Autodesk Inventor part; units mm, degrees
ref_plane "YZ Plane" through (0, 0, 0) normal (1, 0, 0) x (0, 1, 0)
ref_plane "XZ Plane" through (0, 0, 0) normal (0, 1, 0) x (-1, 0, 0)
ref_plane "XY Plane" through (0, 0, 0) normal (0, 0, 1) x (1, 0, 0)
sketch "スケッチ1" plane through (0, 0, 0) normal (1, 0, 0) x (0, 1, 0)
  line L0 (0, 0) -> (0, 6)
  line L1 (0, 6) -> (0, -6)
  line L2 (0, 0) -> (11.5, 0)
  line L3 (11.5, 0) -> (11.5, 9.5)
  line L4 (11.5, 9.5) -> (11.5, -9.5)
  circle A0 centre (0, 6) radius 1.25
  circle A1 centre (0, -6) radius 1.25
  circle A2 centre (11.5, 9.5) radius 1.65
  circle A3 centre (11.5, -9.5) radius 1.65
  circle A4 centre (11.5, 9.5) radius 2.5
  circle A5 centre (11.5, -9.5) radius 2.5
  circle A6 centre (0, 0) radius 2.65
  line L5 (0, 0) -> (-14.6, 0)
  circle A7 centre (-14.6, 0) radius 1.65
  circle A8 centre (-14.6, 0) radius 2.5
  circle A9 centre (0, 6) radius 2
  circle A10 centre (0, -6) radius 2
  line L6 (0, 8) -> (10.6499, 11.851)
  line L7 (0, -8) -> (10.6499, -11.851)
  line L8 (-14.6, 0) -> (-14.6, -2.5)
  line L9 (-14.6, 0) -> (-12.1, 0) construction
  line L10 (-14.6, -2.5) -> (-14.6, 2.5)
  line L11 (-14.6, -2.5) -> (-0.7212, -7.8655)
  line L12 (-14.6, 2.5) -> (-0.7212, 7.8655)
  circle A11 centre (11.5, -9.5) radius 14.9164
  line L13 (11.5, -9.5) -> (0, 0)
  line L14 (11.5, -9.5) -> (0, -2.65)
  line L15 (14, 9.5) -> (14, 6.6979)
  circle A12 centre (11.5, -9.5) radius 16.7294
  circle A13 centre (0, 0) radius 3.575
  circle A14 centre (11.5, -9.5) radius 17.4128
  line L16 (0, 3.575) -> (11.5, 3.575)
  line L17 (0, -3.575) -> (1.5529, -3.575)
  line L18 (3.575, 0) -> (3.575, -4.7795)
  line L19 (1.5529, -3.575) -> (3.575, -3.575)
  circle A15 centre (11.5, -9.5) radius 9.895
  point P0 (9.3522, -8.2206)
  point P1 (0, 2.65)
  point P2 (12.4812, 7.2006)
  point P3 (1.2029, -3.3665)
  point P4 (1.0637, 3.575)
  point P5 (2.9988, -4.4363)
  dimension "d9" = 5
  dimension "d10" = 5.3
  dimension "d0" = 6
  dimension "d1" = 12
  dimension "d2" = 11.5
  dimension "d3" = 9.5
  dimension "d4" = 19
  dimension "d5" = 2.5
  dimension "d6" = 3.3
  dimension "d7" = 3.3
  dimension "d8" = 5
  dimension "d11" = 14.6
  dimension "d12" = 3.3
  dimension "d13" = 5
  dimension "d14" = 4
  dimension "d15" = 4
  dimension "d16" = 90
  dimension "d21" = 7.15
extrude "押し出し2" add sketch "スケッチ1" along normal blind 3 contours A13 L5 A8 L12 A9 L0 | L0 A9 A14 | A14 A9 A4 A12 L16 | L17 L14 A15 L7 A10 L1 | L1 A10 L11 A11 A13 | A11 L11 A12 A13 | A9 A14 | A13 A14 L11 A8 L5 | A14 A9 | A10 | L19 A15 L14 | A12 L11 A14 A13 | A8 L8 A7 L5 | L5 A7 L10 A8 | A9 L6 A4 A14 | A4 A14 A2 L3 A12 | A15 L18 L14 | L14 A5 L7 A15 | L10 A7 L8 A8 | A4 A14 A2 | L3 A2 A14 A4 A12 | A5 L14 A3 L4 | L4 A3 L13 A5 | L13 A3 L14 A5
sketch "スケッチ2" plane through (3, 0, 0) normal (1, 0, 0) x (0, 0, -1)
  point P0 (0, 0)
properties part number "ikafly2b7"
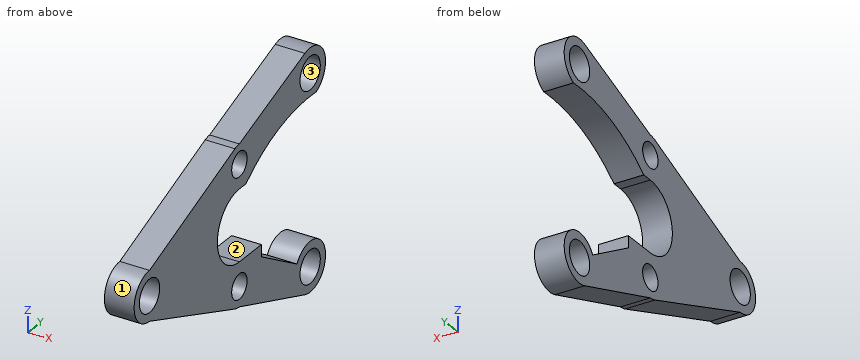
Part model, mm, in its own coordinate system. Face numbers are marked on the shaded views. Coordinates: 2 decimals unless noted, no trailing zeros. Loops run counter-clockwise (first coordinate to the right, second up) from the corner with the lowest first, then second, coordinate; pieces in that order, holes last. Notation, with made-up numbers: (75.5, 87) - (129.5, 87) arc R33 ccw to (129.5, 115) - close; hole circle Ø9 at (-28.75, 82). An arc over 180 degrees is marked (long way). Write each question's results on one line, items separated by ' | '. Start each with the question number.
Q1. Two-plate mould, pull along Y, no slides. Class the marked faces 1, 2 and 3: +Y half, -Y half, draft (parallel to the pull), parting line (faces both ways), or undercut.
Q2. Slice it at D-D on x = 2.05. Give the number of separate pieces and of enclosed holes in the cut face, and give its area (3 significant figures).
Q3. Drop flat-ended pins along their axis: pin 1 Ø5.5 at (y, z) = (-14.6, 0) entering from -X; pin 2 Ø1.5 at (x, y) = (1, 4.5) entering from -Z; pin 3 Ø1.5 at (x, y) = (1.5, 2) entering from +Z; pin 4 Ø0.5 at (x, y) = (1.5, 0.5) entering from -Z. Give the stop position or say it passes through.
Q4. Slice it at B-B on y = -2.5. Give the cut face in (x, z).
Q5. Slice it at C-C on y = 11.5. Give the cut face in (x, z), and give its area (3 significant figures).
Q6. Probe line 1 along Z through (x, y) = (1.05, 11.5); line 2 along Z through (x, y) = (1.1, 0) (3 decimals); line 3 along Z through (x, y) = (1.3, -14.6). List the from-to ranges inside material, lowest first.
Q7. Slice it at A-A on z = 0. Give the cut face in (x, y) (3 decimals).
Answer:
1) face 1: -Y half | face 2: draft | face 3: undercut
2) separate pieces: 1 | enclosed holes: 5 | area: 228 mm2
3) pin 1: stops at x = 0 | pin 2: stops at z = -9.9 | pin 3: stops at z = 8.99 | pin 4: stops at z = -8.27
4) outline: (0, -7.18) - (3, -7.18) - (3, -2.56) - (0, -2.56) - close; (0, 2.56) - (3, 2.56) - (3, 7.18) - (0, 7.18) - close
5) outline: (0, -12) - (3, -12) - (3, -11.15) - (0, -11.15) - close; (0, -7.85) - (3, -7.85) - (3, -7) - (0, -7) - close; (0, 7.23) - (3, 7.23) - (3, 7.85) - (0, 7.85) - close; (0, 11.15) - (3, 11.15) - (3, 12) - (0, 12) - close | area: 9.51 mm2
6) line 1: z = -12 to -11.15, -7.85 to -7, 7.23 to 7.85, 11.15 to 12 | line 2: z = -8 to -7.25, -4.75 to -3.575, 3.575 to 4.75, 7.25 to 8 | line 3: z = -2.5 to -1.65, 1.65 to 2.5
7) outline: (0, -17.1) - (3, -17.1) - (3, -16.25) - (0, -16.25) - close; (0, -12.95) - (3, -12.95) - (3, -3.575) - (0, -3.575) - close
